Here's how the part is built. I have some questions about the finished solid (model axes, mm). A direction names the side the tool comes from. Give positions to 0.01 mm unless a question says otherwise; leave off trailing zeros. Order: outer loops, then holes, each group sorted by start corner. A loop starts at its lowest first (then second) coordinate and runs counter-clockwise, first axis right, second up. Notation, with made-up numbers: (-23.5, -8.5) -> (14.5, -8.5) arc R11 cw to (14.5, 4.5) -> close; hole circle Ø3 at (-34, 89). An arc over 180 degrees is marked (long way). Write each question's results on one line, items separated by ' | '. Start each with the question number.
Q1. Imagine slicing it at A-A, the plane y = -0.5. Please give me the cut outline in (x, z).
Q2. Imagine slicing it at D-D, the plane y = 1.5. Please give me the cut outline in (x, z), then the cut area to 3 significant figures.
Q3. I'm going to push a flat-ended pin straight in: pin 1 (5 mm diameter, centred on x = -6, z = -1.5, fed in from -Y). Where does the tip first touch, or does it pass through?
Q4. For faces 4 (the face through (15.5, -1, 0)), 5 (the face through (0, 1, 8)), 6 (the face through (18.7, 1, 0)), which set-ups out of +Z, -Z, +X, -X, +Y, -Y let a thin tool reach every point of the face, with its end or its side?
Q5. Thinking about a two-plate mould opening in X: for faces 1 (the face through (-15.5, -1, 0)), 2 (the face through (19, -1.2, 0)), 3 (the face through (-20, 1, 0)), which applies, pulls with the +X half, pulls with the -X half, needs draft (parallel to the pull), parting line crosses it, or undercut?
Q6. Imagine slicing it at B-B, the plane x = -17.75. Please give me the cut outline in (y, z).
Q7. Imagine slicing it at C-C, the plane z = 5. Please give me the cut outline in (x, y).
Q8. I need wall thicknesses on line 1 along X through (y, z) = (-0.55, 0.25); line 2 along X through (y, z) = (2.2, 0); line 3 along X through (y, z) = (0.5, 1.6). Which ranges of each line are inside material? Lowest first, please. Write a range as [from, to].
```python
from build123d import *

# Parameters (mm, degrees)
SKETCH1_W           = 40
SKETCH1_H           = 16
BOSS_EXTRUDE1_DEPTH = 2.5
SKETCH2_W           = 4.5
SKETCH2_H           = 16
BOSS_EXTRUDE2_DEPTH = 1.2
CUT_EXTRUDE1_DEPTH  = 4.7
SKETCH4_R           = 0.95
CUT_EXTRUDE2_DEPTH  = 4.7


with BuildPart() as part:
    # Sketch1 → Boss-Extrude1 (new body)
    with BuildSketch(Plane(origin=(0, 0, 0), x_dir=(1, 0, 0), z_dir=(0, 1, 0))):
        Rectangle(SKETCH1_W, SKETCH1_H)
    extrude(amount=BOSS_EXTRUDE1_DEPTH)

    # Sketch2 → Boss-Extrude2 (add)
    with BuildSketch(Plane.XZ):
        with Locations((-17.75, 0)):
            Rectangle(SKETCH2_W, SKETCH2_H)
    boss_extrude2 = extrude(amount=BOSS_EXTRUDE2_DEPTH)

    # Sketch3 → Cut-Extrude1 (cut, through all)
    with BuildSketch(Plane.XZ.offset(1.2)):
        with BuildLine():
            Line((-16.8, 5.5), (-16.8, -5.5))
            ThreePointArc((-16.8, -5.5), (-17.75, -6.45), (-18.7, -5.5))
            Line((-18.7, -5.5), (-18.7, 5.5))
            ThreePointArc((-18.7, 5.5), (-17.75, 6.45), (-16.8, 5.5))
        make_face()
    cut_extrude1 = extrude(amount=-CUT_EXTRUDE1_DEPTH, mode=Mode.SUBTRACT)

    # Mirror1: Boss-Extrude2, Cut-Extrude1 across plane
    add(boss_extrude2.mirror(Plane(origin=(0, 0, 0), x_dir=(0, 0, 1), z_dir=(1, 0, 0))))
    add(cut_extrude1.mirror(Plane(origin=(0, 0, 0), x_dir=(0, 0, 1), z_dir=(1, 0, 0))), mode=Mode.SUBTRACT)

    # Sketch4 → Cut-Extrude2 (cut, through all)
    with BuildSketch(Plane(origin=(0, 2.5, 0), x_dir=(1, 0, 0), z_dir=(0, 1, 0))):
        with Locations((4.25, -1.6)):
            Circle(SKETCH4_R)
        with Locations((-4.25, -1.6)):
            Circle(SKETCH4_R)
        with Locations((0, 6)):
            Circle(SKETCH4_R)
    extrude(amount=-CUT_EXTRUDE2_DEPTH, mode=Mode.SUBTRACT)


solid = part.part
```
Geometry check:
1) outline: (-20, -8) -> (-15.5, -8) -> (-15.5, 8) -> (-20, 8) -> close; (15.5, -8) -> (20, -8) -> (20, 8) -> (15.5, 8) -> close; hole (-18.7, -5.5) arc R0.95 ccw to (-16.8, -5.5) -> (-16.8, 5.5) arc R0.95 ccw to (-18.7, 5.5) -> close; hole (16.8, -5.5) arc R0.95 ccw to (18.7, -5.5) -> (18.7, 5.5) arc R0.95 ccw to (16.8, 5.5) -> close
2) outline: (-20, -8) -> (20, -8) -> (20, 8) -> (-20, 8) -> close; hole (-18.7, -5.5) arc R0.95 ccw to (-16.8, -5.5) -> (-16.8, 5.5) arc R0.95 ccw to (-18.7, 5.5) -> close; hole circle Ø1.9 at (-4.25, 1.6); hole circle Ø1.9 at (0, -6); hole circle Ø1.9 at (4.25, 1.6); hole (16.8, -5.5) arc R0.95 ccw to (18.7, -5.5) -> (18.7, 5.5) arc R0.95 ccw to (16.8, 5.5) -> close | area: 584 mm²
3) pin 1: y = 0
4) face 4: +Z, -Z, -Y | face 5: +Z, +X, -X, +Y, -Y | face 6: +Y, -Y
5) face 1: undercut | face 2: needs draft | face 3: pulls with the -X half
6) outline: (-1.2, -8) -> (2.5, -8) -> (2.5, -6.45) -> (-1.2, -6.45) -> close; (-1.2, 6.45) -> (2.5, 6.45) -> (2.5, 8) -> (-1.2, 8) -> close
7) outline: (-20, -1.2) -> (-18.7, -1.2) -> (-18.7, 2.5) -> (-20, 2.5) -> close; (-16.8, -1.2) -> (-15.5, -1.2) -> (-15.5, 0) -> (15.5, 0) -> (15.5, -1.2) -> (16.8, -1.2) -> (16.8, 2.5) -> (-16.8, 2.5) -> close; (18.7, -1.2) -> (20, -1.2) -> (20, 2.5) -> (18.7, 2.5) -> close
8) line 1: [-20, -18.7], [-16.8, -15.5], [15.5, 16.8], [18.7, 20] | line 2: [-20, -18.7], [-16.8, 16.8], [18.7, 20] | line 3: [-20, -18.7], [-16.8, -5.2], [-3.3, 3.3], [5.2, 16.8], [18.7, 20]
